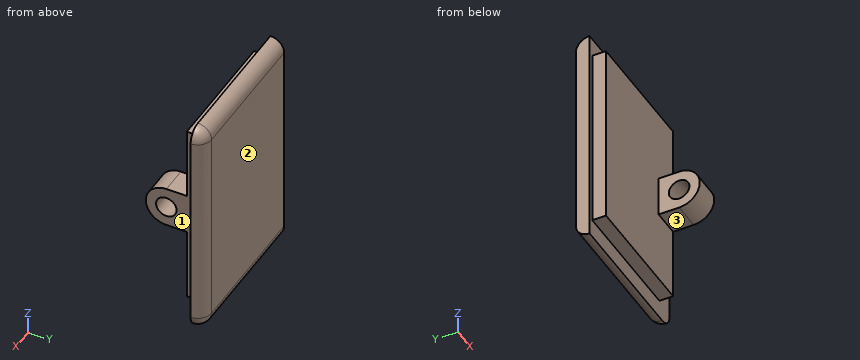
```python
from build123d import *

# Parameters (mm, degrees)
SKETCH1_W           = 18.5
SKETCH1_H           = 27.5
BOSS_EXTRUDE1_DEPTH = 2
SKETCH3_R           = 1.5
BOSS_EXTRUDE2_DEPTH = 4
BOSS_EXTRUDE3_DEPTH = 2
FILLET1_R           = 2


with BuildPart() as part:
    # Sketch1 → Boss-Extrude1 (new body)
    with BuildSketch(Plane(origin=(0, 0, 0), x_dir=(1, 0, 0), z_dir=(0, 1, 0))):
        with Locations((-10, 14.5)):
            Rectangle(SKETCH1_W, SKETCH1_H)
    extrude(amount=-BOSS_EXTRUDE1_DEPTH)

    # Sketch3 → Boss-Extrude2 (add)
    with BuildSketch(Plane(origin=(-0.75, 0, 0), x_dir=(0, 0, -1), z_dir=(1, 0, 0))):
        with BuildLine():
            Line((11.5, -5), (11.5, -2))
            Line((11.5, -2), (17.5, -2))
            Line((17.5, -2), (17.5, -5))
            ThreePointArc((17.5, -5), (14.5, -8), (11.5, -5))
        make_face()
        with Locations((14.5, -5)):
            Circle(SKETCH3_R, mode=Mode.SUBTRACT)
    extrude(amount=-BOSS_EXTRUDE2_DEPTH)

    # Sketch4 → Boss-Extrude3 (add)
    with BuildSketch(Plane(origin=(0, 0, 0), x_dir=(1, 0, 0), z_dir=(0, 1, 0))):
        with BuildLine():
            Line((0, -2), (-20, -2))
            Line((-20, -2), (-20, 31))
            Line((-20, 31), (0, 31))
            ThreePointArc((0, 31), (1.414213562, 30.414213562), (2, 29))
            Line((2, 29), (2, 0))
            ThreePointArc((2, 0), (1.414213562, -1.414213562), (0, -2))
        make_face()
    extrude(amount=BOSS_EXTRUDE3_DEPTH)

    # Fillet1
    fillet1_edges = [part.edges().sort_by_distance(p)[0] for p in [
        (-10, 2, -31),
        (1.414213562, 2, -30.414213562),
        (2, 2, -14.5),
        (1.414213562, 2, 1.414213562),
        (-10, 2, 2),
    ]]
    fillet(fillet1_edges, radius=FILLET1_R - 0.0001)  # a hair under: the kernel refuses the full size


solid = part.part
```
Geometry: final body of the model. Coordinates: model frame, mm. Face numbers are marked on the shaded views. A direction names the side the tool comes from. Round coordinates to 2 decimals unless told otherwise and drop trailing zeros. Use one line per item in the form item = value. Start each with the question number.
1. Line query: probe 1 along Y at (x, z) = (-3.75, -14.5); probe 2 along Z at (x, y) = (-14, -1.25); probe 3 along Y at (x, z) = (-16, -9.5). Output: solid intervals per line, ascending.
2. Reachability of the marked faces 1, 2 and 3 from +Z, -Z, +X, -X, +Y, -Y: full face, straight path, thin tool, end or side. Return the list, or none.
3. Pin query (flat end, axial travel): pin 1 Ø6 at (x, y) = (-6.5, -4.5) entering from +Z; pin 2 Ø3 at (y, z) = (-6, -15) entering from -X; pin 3 Ø0.6 at (y, z) = (-1.5, -8.5) entering from -X. Return the tip coordinate at first contact, or that it passes through.
Solution:
q1.probe_1 = -8 to -6.5, -3.5 to 2
q1.probe_2 = -28.25 to -0.75
q1.probe_3 = -2 to 2
q2.face_1 = +Z, -Z, +X, -Y
q2.face_2 = +Z, -Z, +X, -X, +Y
q2.face_3 = -Z, +X, -X, -Y
q3.pin_1 = -0.75
q3.pin_2 = -4.75
q3.pin_3 = -19.25
